Part model, mm, in its own coordinate system. A direction names the side the tool comes from. Coordinates: 2 decimals unless noted, no trailing zeros. Order: outer loops, then holes, each group sorted by start corner. A loop starts at its lowest first (then second) coordinate and runs counter-clockwise, first axis right, second up.
from build123d import *

# Parameters (mm, degrees)
SKETCH3_R                = 7.5
BOSS_EXTRUDE1_DEPTH      = 22
BOSS_EXTRUDE2_DEPTH      = 10
BOSS_EXTRUDE2_DEPTH_BACK = 10
SKETCH1_R                = 12.5
SKETCH6_R                = 10.005
CUT_EXTRUDE1_DEPTH       = 49
SKETCH5_R                = 5.005
CUT_EXTRUDE2_DEPTH       = 15


with BuildPart() as part:
    # Sketch3 → Boss-Extrude1 (new body)
    with BuildSketch(Plane(origin=(0, 30, 0), x_dir=(1, 0, 0), z_dir=(0, 1, 0))):
        with Locations(Location((0, 0, 0), (0, 0, 270))):
            Circle(SKETCH3_R)
    extrude(amount=-BOSS_EXTRUDE1_DEPTH)

    # Sketch1 → Boss-Extrude2 (add, two sides: drawn at the far end of the back side and taken through both)
    with BuildSketch(Plane.XY.offset(-BOSS_EXTRUDE2_DEPTH_BACK)):
        Circle(SKETCH1_R)
    extrude(amount=BOSS_EXTRUDE2_DEPTH + BOSS_EXTRUDE2_DEPTH_BACK)

    # Sketch6 → Cut-Extrude1 (cut)
    with BuildSketch(Plane(origin=(0, 0, -10), x_dir=(-1, 0, 0), z_dir=(0, 0, -1))):
        Circle(SKETCH6_R)
    extrude(amount=-CUT_EXTRUDE1_DEPTH, mode=Mode.SUBTRACT)

    # Sketch5 → Cut-Extrude2 (cut)
    with BuildSketch(Plane(origin=(0, 30, 0), x_dir=(1, 0, 0), z_dir=(0, 1, 0))):
        with Locations(Location((0, 0, 0), (0, 0, 270))):
            Circle(SKETCH5_R)
    extrude(amount=-CUT_EXTRUDE2_DEPTH, mode=Mode.SUBTRACT)


solid = part.part
Q1. Wall check: line 1 along X through (y, z) = (23.75, 0) (3 decimals); line 2 along Y through (x, z) = (0, 5.75) (3 decimals); line 3 along Y through (x, z) = (0, 1.25) (3 decimals). Give the ranges that are in metal, low to high.
Results list:
line 1: x = -7.5 to -5.005, 5.005 to 7.5
line 2: y = -12.5 to -10.005, 10.005 to 30
line 3: y = -12.5 to -10.005, 10.005 to 15
Q2. Cut at A-A on z = 0. Write the cut outline in (x, y) (3 decimals), and give its area (3 significant figures).
Results list:
outline: (-7.5, 10) arc R12.5 ccw (long way) to (7.5, 10) - (7.5, 30) - (5.005, 30) - (5.005, 15) - (-5.005, 15) - (-5.005, 30) - (-7.5, 30) - close; hole circle Ø20.01 at (0, 0)
area: 301 mm2
Q3. Cut at C-C on y = 0. Write the cut outline in (x, z) (3 decimals), and give its area (3 significant figures).
Results list:
outline: (-12.5, -10) - (-10.005, -10) - (-10.005, 10) - (-12.5, 10) - close; (10.005, -10) - (12.5, -10) - (12.5, 10) - (10.005, 10) - close
area: 99.8 mm2
Q4. Pin check, flat tips, straight feed: pin 1 Ø2 at (x, z) = (-8.5, 3.5) entering from -Y; pin 2 Ø8 at (y, z) = (18.5, -1) entering from +X; pin 3 Ø3 at (x, z) = (-0.5, 1.5) entering from +Y. Stop position of each tip, or through.
Results list:
pin 1: stops at y = -10
pin 2: stops at x = 7.5
pin 3: stops at y = 15
Q5. Mould opens along X. For faces 3 (the face through (2.169, -9.767, -0.14)), 4 (the face through (-2.71, -12.203, -0.14)), 5 (the face through (0, 15, 0)), 6 (the face through (-0.1, 10.2, 10)) say: pulls with the +X half, pulls with the -X half, needs draft (parallel to the pull), parting line crosses it, or undercut.
Results list:
face 3: undercut
face 4: parting line crosses it
face 5: undercut
face 6: needs draft
Q6. Which spindle directions (+Z, -Z, +X, -X, +Y, -Y) get a long thin tool onto all of the face, cutting with end or side? Do faces 1 (the face through (-0.1, 10.2, -10)), 2 (the face through (-3.05, 22.6, -3.97)). Say none if no direction does.
Results list:
face 1: -Z, +X, -X, +Y, -Y
face 2: +Y
Q7. Cut at B-B on x = 0. Write the cut outline in (y, z) (3 decimals), and give its area (3 significant figures).
Results list:
outline: (-12.5, -10) - (-10.005, -10) - (-10.005, 10) - (-12.5, 10) - close; (10.005, -10) - (12.5, -10) - (12.5, -7.5) - (30, -7.5) - (30, -5.005) - (15, -5.005) - (15, 5.005) - (30, 5.005) - (30, 7.5) - (12.5, 7.5) - (12.5, 10) - (10.005, 10) - close
area: 212 mm2
Q8. Cut at D-D on y = 20. Write the cut outline in (x, z) (3 decimals), and give its area (3 significant figures).
Results list:
outline: circle Ø15 at (0, 0); hole circle Ø10.01 at (0, 0)
area: 98.0 mm2
